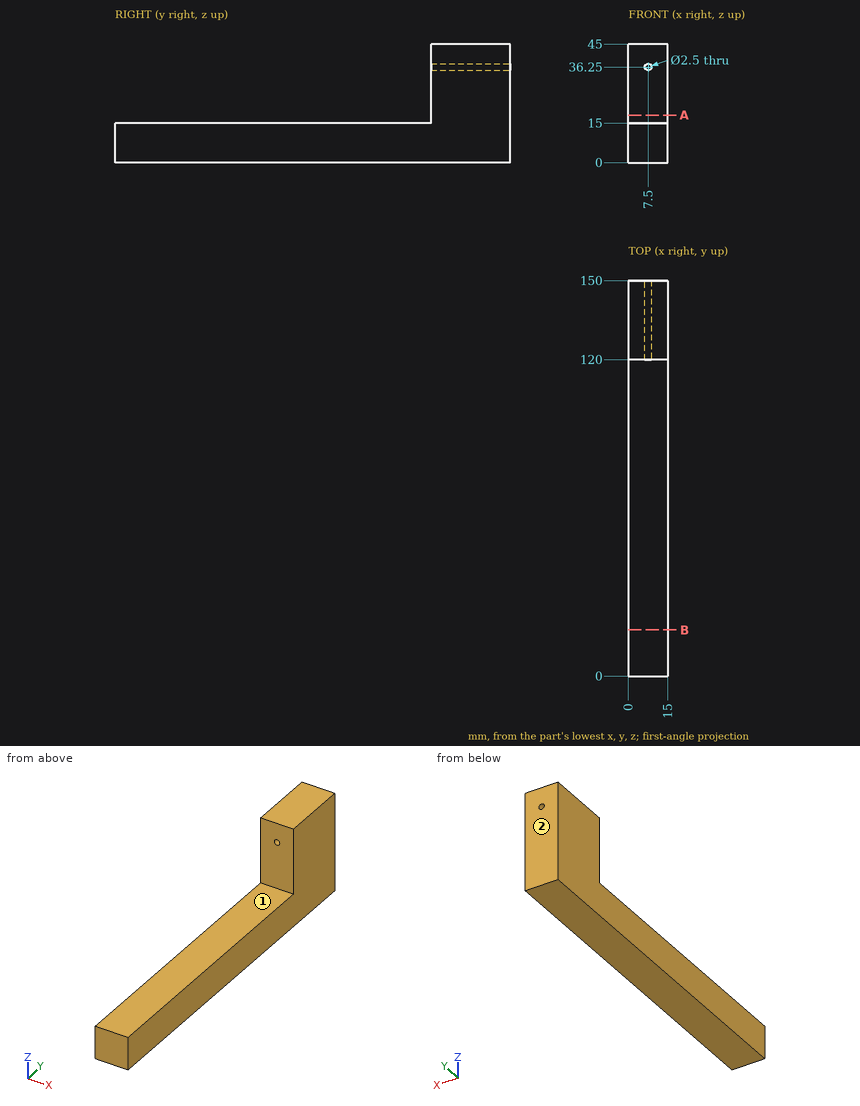
Source: three-view drawing plus pictorial views. Frame: mm from the lowest corner of the part. A direction names the side the tool comes from. Give positions to 0.01 mm unless a question says otherwise; leave off trailing zeros. Order: outer loops, then holes, each group sorted by start corner. A loop starts at its lowest first (then second) coordinate and runs counter-clockwise, first axis right, second up. Notation, with made-up numbers: M 46.25,-37 L 98.25,-37 A19 ccw 98.25,-11 Z; hole C 48,48 d2. An arc over 180 degrees is marked long. Return JSON: item names as keys, results as strings.
1) Contact query for flat-ended pins moving along their axis: pin 1 (5 mm diameter, centred on y = 121, z = 35.5, fed in from -X); pin 2 (1.5 mm diameter, centred on x = 4.5, y = 42, fed in from +Z); pin 3 (5 mm diameter, centred on y = 110, z = 18, fed in from -X). Output: stop coordinate, or through.
Taken from the geometry:
{"pin 1": "stops at x = 0", "pin 2": "stops at z = 15", "pin 3": "passes through"}
2) Section query A-A on z = 18. Output: boundary loops of the cut face in (x, y).
Taken from the geometry:
{"outline": "M 0,120 L 15,120 L 15,150 L 0,150 Z"}
3) Line query: L1, parallel to X at y = 141, z = 36.25; L2, parallel to Z at x = 7.5, y = 143.25; L3, parallel to Z at x = 9.75, y = 34. Output: solid intervals per line, ascending. Write a range as [from, to].
Taken from the geometry:
{"L1": "x = [0, 6.25], [8.75, 15]", "L2": "z = [0, 35], [37.5, 45]", "L3": "z = [0, 15]"}
4) Section query B-B on y = 17.5. Output: boundary loops of the cut face in (x, z).
Taken from the geometry:
{"outline": "M 0,0 L 15,0 L 15,15 L 0,15 Z"}
5) Access query for the marked faces 1 and 2. Directions: +Z, -Z, +X, -X, +Y, -Y. A direction counts if a zero-diameter tool reaches every point of the face in a straight line with its end or side. Return the directions, or none.
Taken from the geometry:
{"face 1": "+Z, +X, -X, -Y", "face 2": "+Z, -Z, +X, -X, +Y"}
